from build123d import *

# Parameters (mm, degrees)
SKETCH1_W           = 40
SKETCH1_H           = 40
BOSS_EXTRUDE1_DEPTH = 15
SKETCH3_R           = 1.75
CUT_EXTRUDE2_DEPTH  = 16
SKETCH4_R           = 3
CUT_EXTRUDE3_DEPTH  = 7
FILLET1_R           = 1
SKETCH5_R           = 12.5
CUT_EXTRUDE4_DEPTH  = 3.5


with BuildPart() as part:
    # Sketch1 → Boss-Extrude1 (new body)
    with BuildSketch(Plane.XY):
        Rectangle(SKETCH1_W, SKETCH1_H)
    extrude(amount=BOSS_EXTRUDE1_DEPTH)

    # Sketch3 → Cut-Extrude2 (cut, through all)
    with BuildSketch(Plane.XY.offset(15)):
        with Locations((15, 15)):
            Circle(SKETCH3_R)
        with Locations((15, -15)):
            Circle(SKETCH3_R)
        with Locations((-15, 15)):
            Circle(SKETCH3_R)
        with Locations((-15, -15)):
            Circle(SKETCH3_R)
    extrude(amount=-CUT_EXTRUDE2_DEPTH, mode=Mode.SUBTRACT)

    # Sketch4 → Cut-Extrude3 (cut)
    with BuildSketch(Plane.XY.offset(15)):
        with Locations((15, 15)):
            Circle(SKETCH4_R)
        with Locations((15, -15)):
            Circle(SKETCH4_R)
        with Locations((-15, -15)):
            Circle(SKETCH4_R)
        with Locations((-15, 15)):
            Circle(SKETCH4_R)
    extrude(amount=-CUT_EXTRUDE3_DEPTH, mode=Mode.SUBTRACT)

    # Fillet1
    fillet1_edges = [part.edges().sort_by_distance(p)[0] for p in [
        (12, 15, 15),
        (12, -15, 15),
        (-18, -15, 15),
        (-18, 15, 15),
    ]]
    fillet(fillet1_edges, radius=FILLET1_R)

    # Sketch5 → Cut-Extrude4 (cut)
    with BuildSketch(Plane.XY.offset(15)):
        Circle(SKETCH5_R)
    extrude(amount=-CUT_EXTRUDE4_DEPTH, mode=Mode.SUBTRACT)


solid = part.part
Build history of the part. All positions in model axes, mm. A direction names the side the tool comes from. Round coordinates to 2 decimals unless told otherwise and drop trailing zeros. Write each loop counter-clockwise with the first axis right and the second up, starting at its lowest first coordinate (ties: lowest second). Pieces come first, ordered by that corner, then holes. Notation, with made-up numbers: (68.5, 38.5) -> (116.5, 38.5) arc R10 cw to (116.5, 49.5) -> close; hole circle Ø7 at (71, 57). An arc over 180 degrees is marked (long way). Write item = value, one per line.
(1) Band-saw the part on B-B (y = 15). Give the cut face in (x, z), then the cut area to 3 significant figures.
Answer:
outline = (-20, 0) -> (-16.75, 0) -> (-16.75, 8) -> (-18, 8) -> (-18, 14) arc R1 ccw to (-19, 15) -> (-20, 15) -> close; (-13.25, 0) -> (13.25, 0) -> (13.25, 8) -> (12, 8) -> (12, 14) arc R1 ccw to (11, 15) -> (-11, 15) arc R1 ccw to (-12, 14) -> (-12, 8) -> (-13.25, 8) -> close; (16.75, 0) -> (20, 0) -> (20, 15) -> (19, 15) arc R1 ccw to (18, 14) -> (18, 8) -> (16.75, 8) -> close
area = 459 mm2
(2) Flat gauge pins, fed straight in: pin 1 (5 mm diameter, centred on x = -16, y = 16, fed in from +Z); pin 2 (2 mm diameter, centred on x = 15, y = -15, fed in from -Z); pin 3 (5.5 mm diameter, centred on x = 15, y = 15, fed in from +Z); pin 4 (1 mm diameter, centred on x = 1.5, y = -9, fed in from -Z). Where does each tip first touch, or does it go through?
Answer:
pin_1 = 15
pin_2 = through
pin_3 = 8
pin_4 = 0
(3) Two-plate mould, pull along Y, no slides. Class faces 1 (the face through (12.6, -16.8, 11)), 2 (the face through (-20, 0, 7)), 3 (the face through (0, -20, 7)): pulls with the +Y half, pulls with the -Y half, needs draft (parallel to the pull), parting line crosses it, or undercut.
Answer:
face_1 = undercut
face_2 = needs draft
face_3 = pulls with the -Y half
(4) Band-saw the part on A-A (z = 12). Give the cut face in (x, y), then the cut area to 3 significant figures.
Answer:
outline = (-20, -20) -> (20, -20) -> (20, 20) -> (-20, 20) -> close; hole circle Ø6 at (-15, -15); hole circle Ø6 at (-15, 15); hole circle Ø25 at (0, 0); hole circle Ø6 at (15, -15); hole circle Ø6 at (15, 15)
area = 996 mm2
(5) Tool access for faces 4 (the face through (0, 0, 11.5)), 5 (the face through (14.772, -13.265, 4.056)): list every direction of +Z, -Z, +X, -X, +Y, -Y with a clear straight run to the whole face (end or side of a thin tool).
Answer:
face_4 = +Z
face_5 = +Z, -Z
(6) Probe L1, parallel to Y at x = 15, z = 10.9; L2, parallel to Y at x = 0, z = 13.95; L3, parallel to Y at x = 15, z = 5.5. List the from-to ranges inside material, lowest first.
Answer:
L1 = -20 to -18, -12 to 12, 18 to 20
L2 = -20 to -12.5, 12.5 to 20
L3 = -20 to -16.75, -13.25 to 13.25, 16.75 to 20
(7) Band-saw the part on D-D (z = 4.5). Give the cut face in (x, y), then the cut area to 3 significant figures.
Answer:
outline = (-20, -20) -> (20, -20) -> (20, 20) -> (-20, 20) -> close; hole circle Ø3.5 at (-15, -15); hole circle Ø3.5 at (-15, 15); hole circle Ø3.5 at (15, -15); hole circle Ø3.5 at (15, 15)
area = 1,560 mm2
